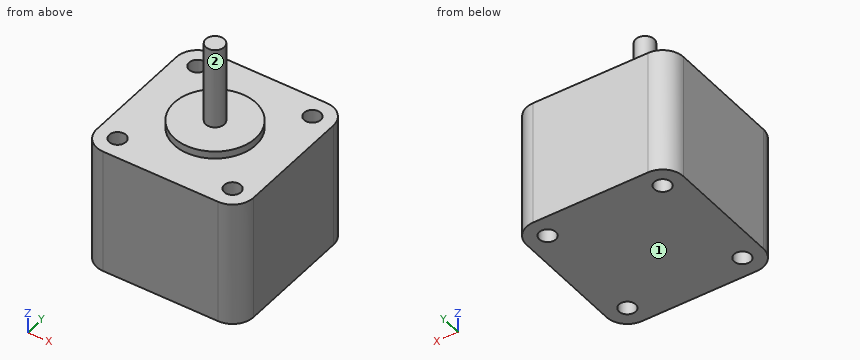
```python
from build123d import *

# Parameters (mm, degrees)
SKETCH1_R           = 2.5
BOSS_EXTRUDE1_DEPTH = 24
SKETCH2_R           = 11
BOSS_EXTRUDE2_DEPTH = 2
BOSS_EXTRUDE3_DEPTH = 34
SKETCH5_R           = 2.25
CUT_EXTRUDE1_DEPTH  = 34


with BuildPart() as part:
    # Sketch1 → Boss-Extrude1 (new body)
    with BuildSketch(Plane.XY):
        Circle(SKETCH1_R)
    extrude(amount=BOSS_EXTRUDE1_DEPTH)

    # Sketch2 → Boss-Extrude2 (add)
    with BuildSketch(Plane.XY):
        Circle(SKETCH2_R)
    extrude(amount=BOSS_EXTRUDE2_DEPTH)

    # Sketch4 → Boss-Extrude3 (add)
    with BuildSketch(Plane(origin=(0, 0, 0), x_dir=(-1, 0, 0), z_dir=(0, 0, -1))):
        with BuildLine():
            Line((15.5, 21.15), (-15.5, 21.15))
            ThreePointArc((-15.5, 21.15), (-19.495153314, 19.495153314), (-21.15, 15.5))
            Line((-21.15, 15.5), (-21.15, -15.5))
            ThreePointArc((-21.15, -15.5), (-19.495153314, -19.495153314), (-15.5, -21.15))
            Line((-15.5, -21.15), (15.5, -21.15))
            ThreePointArc((15.5, -21.15), (19.495153314, -19.495153314), (21.15, -15.5))
            Line((21.15, -15.5), (21.15, 15.5))
            ThreePointArc((21.15, 15.5), (19.495153314, 19.495153314), (15.5, 21.15))
        make_face()
    extrude(amount=BOSS_EXTRUDE3_DEPTH)

    # Sketch5 → Cut-Extrude1 (cut)
    with BuildSketch(Plane(origin=(0, 0, -34), x_dir=(-1, 0, 0), z_dir=(0, 0, -1))):
        with Locations((-15.5, -15.5)):
            Circle(SKETCH5_R)
        with Locations(Location((15.5, -15.5, 0), (0, 0, 180))):
            Circle(SKETCH5_R)
        with Locations(Location((-15.5, 15.5, 0), (0, 0, 180))):
            Circle(SKETCH5_R)
        with Locations((15.5, 15.5)):
            Circle(SKETCH5_R)
    extrude(amount=-CUT_EXTRUDE1_DEPTH, mode=Mode.SUBTRACT)


solid = part.part
```
Build history of the part. All positions in model axes, mm. Face numbers are marked on the shaded views. A direction names the side the tool comes from. Coordinates: 2 decimals unless noted, no trailing zeros. Order: outer loops, then holes, each group sorted by start corner. A loop starts at its lowest first (then second) coordinate and runs counter-clockwise, first axis right, second up. Notation, with made-up numbers: M -7,-1 L 14,-1 A27 ccw 14,16 Z; hole C -1.75,-19 d3. An arc over 180 degrees is marked long. One line per question, with ' | ' between items. Start each with the question number.
1. Cut at B-B (z = -18). Write the cut outline in (x, y), plus the area to 3 significant figures.
2. Flat gauge pins, fed straight in: P1, Ø3.5, axis at x = -15.5, y = -15.5, coming from the -Z side; P2, Ø6, axis at x = 15.5, y = -15.5, coming from the +Z side; P3, Ø10, axis at x = 1, y = 8.5, coming from the +Z side. Where does each tip first touch, or does it go through?
3. Wall check: line 1 along Y through (x, z) = (-15.5, -22); line 2 along X through (y, z) = (17.5, -24.5); line 3 along X through (y, z) = (-16, -31). Give the ranges that are in metal, low to high. Write a range as [from, to].
4. Cut at C-C (x = 17). Write the cut outline in (y, z), plus the area to 3 significant figures.
5. Cut at D-D (x = -7). Write the cut outline in (y, z), plus the area to 3 significant figures.
6. Tool access for the marked faces 1 and 2: list every direction of +Z, -Z, +X, -X, +Y, -Y with a clear straight run to the whole face (end or side of a thin tool).
7. Cut at A-A (y = 16.5). Write the cut outline in (x, z), plus the area to 3 significant figures.
The answers:
1) outline: M -21.15,-15.5 A5.65 ccw -15.5,-21.15 L 15.5,-21.15 A5.65 ccw 21.15,-15.5 L 21.15,15.5 A5.65 ccw 15.5,21.15 L -15.5,21.15 A5.65 ccw -21.15,15.5 Z; hole C -15.5,-15.5 d4.5; hole C -15.5,15.5 d4.5; hole C 15.5,-15.5 d4.5; hole C 15.5,15.5 d4.5 | area: 1,700 mm2
2) P1: passes through | P2: stops at z = 0 | P3: stops at z = 2
3) line 1: y = [-21.15, -17.75], [-13.25, 13.25], [17.75, 21.15] | line 2: x = [-20.78, -16.53], [-14.47, 14.47], [16.53, 20.78] | line 3: x = [-21.13, -17.69], [-13.31, 13.31], [17.69, 21.13]
4) outline: M -20.95,-34 L -17.18,-34 L -17.18,0 L -20.95,0 Z; M -13.82,-34 L 13.82,-34 L 13.82,0 L -13.82,0 Z; M 17.18,-34 L 20.95,-34 L 20.95,0 L 17.18,0 Z | area: 1,200 mm2
5) outline: M -21.15,-34 L 21.15,-34 L 21.15,0 L 8.49,0 L 8.49,2 L -8.49,2 L -8.49,0 L -21.15,0 Z | area: 1,470 mm2
6) face 1: -Z, +X, -X, +Y, -Y | face 2: +Z
7) outline: M -21.06,-34 L -17.52,-34 L -17.52,0 L -21.06,0 Z; M -13.48,-34 L 13.48,-34 L 13.48,0 L -13.48,0 Z; M 17.52,-34 L 21.06,-34 L 21.06,0 L 17.52,0 Z | area: 1,160 mm2
